```python
from build123d import *

# Parameters (mm, degrees)
F0_R           = 4.7625
F1_DEPTH       = 19.05
F2_R           = 1.8288
F3_DEPTH       = 2.38125
F4_R           = 1.35255
F5_DEPTH       = 2.38125
F8_DEPTH       = 1.190625
F9_R           = 5.55625
F9_R_2         = 4.7625
F11_DEPTH      = 0.79375
F11_DEPTH_BACK = 19.84375
F12_R          = 1.7272
F13_DEPTH      = 10.0554862042
F15_DEPTH      = 19.05
F16_R          = 2.15265
F17_DEPTH      = 2.38125
F18_R          = 1.190625


with BuildPart() as f1:
    # F0 (on Top) → F1 (new body)
    with BuildSketch(Plane.XY):
        Polygon((-12.7, -13.49375), (12.7, -13.49375), (12.7, -21.43125), (15.08125, -21.43125), (15.08125, -11.1125), (7.14375, -11.1125), (7.14375, 7.3428228204), (2.38125, 7.7594875805), (2.38125, 7.14375), (-2.38125, 7.14375), (-2.38125, 7.7594875805), (-7.14375, 7.3428228204), (-7.14375, -11.1125), (-15.08125, -11.1125), (-15.08125, -21.43125), (-12.7, -21.43125), align=None)
        Circle(F0_R, mode=Mode.SUBTRACT)
    extrude(amount=F1_DEPTH)

    # F2 (on face) → F3 (cut, through all)
    with BuildSketch(Plane.YZ.offset(15.08125)):
        with Locations((-18.25625, 15.875)):
            Circle(F2_R)
        with Locations((-18.25625, 3.175)):
            Circle(F2_R)
    extrude(amount=-F3_DEPTH, mode=Mode.SUBTRACT)

    # F4 (on face) → F5 (cut, through all)
    with BuildSketch(Plane(origin=(-15.08125, 0, 0), x_dir=(0, -1, 0), z_dir=(-1, 0, 0))):
        with Locations((18.25625, 3.175)):
            Circle(F4_R)
        with Locations((18.25625, 15.875)):
            Circle(F4_R)
    extrude(amount=-F5_DEPTH, mode=Mode.SUBTRACT)

    # F7 (on offset) → F8 (join, symmetric)
    with BuildSketch(Plane(origin=(0, 0, 9.525), x_dir=(1, 0, 0), z_dir=(0, 0, -1))):
        Polygon((-15.08125, 11.1125), (-7.14375, -7.3428228204), (-7.14375, 11.1125), align=None)
        Polygon((15.08125, 11.1125), (7.14375, 11.1125), (7.14375, -7.3428228204), align=None)
    extrude(amount=F8_DEPTH, both=True)

    # F9 (on face) → F11 (join, two sides)
    with BuildSketch(Plane(origin=(0, 0, 0), x_dir=(1, 0, 0), z_dir=(0, 0, -1))) as f11_sk:
        Circle(F9_R)
        Circle(F9_R_2, mode=Mode.SUBTRACT)
    extrude(amount=F11_DEPTH)
    extrude(f11_sk.sketch, amount=-F11_DEPTH_BACK)

    # F12 (on face) → F13 (cut, up to face)
    with BuildSketch(Plane.XZ.offset(13.49375)):
        with Locations((0, 9.525)):
            Circle(F12_R)
    extrude(amount=-F13_DEPTH, mode=Mode.SUBTRACT)

    # F14 (on face) → F15 (cut, through all)
    with BuildSketch(Plane.XY.offset(19.05)):
        with BuildLine():
            Line((-4.7625, -5.3246368714), (-4.7625, -11.1125))
            Line((-4.7625, -11.1125), (4.7625, -11.1125))
            Line((4.7625, -11.1125), (4.7625, -5.3246368714))
            ThreePointArc((4.7625, -5.3246368714), (0, -7.14375), (-4.7625, -5.3246368714))
        make_face()
    extrude(amount=-F15_DEPTH, mode=Mode.SUBTRACT)

    # F16 (on face) → F17 (cut, through all)
    with BuildSketch(Plane.XZ.offset(13.49375)):
        with Locations((0, 9.525)):
            Circle(F16_R)
    extrude(amount=-F17_DEPTH, mode=Mode.SUBTRACT)

    # F18
    f18_edges = [f1.edges().sort_by_distance(p)[0] for p in [
        (7.14375, -11.1125, 4.167187),
        (7.14375, -11.1125, 14.882812),
        (-7.14375, -11.1125, 4.167187),
        (-7.14375, -11.1125, 14.882812),
        (-4.7625, -11.1125, 9.525),
        (4.7625, -11.1125, 9.525),
        (4.7625, -5.324637, 9.525),
        (-4.7625, -5.324637, 9.525),
    ]]
    fillet(f18_edges, radius=F18_R)


solid = f1.part
```
Check sheet for the modelled part. Datum: model origin and axes. Units: mm. A direction names the side the tool comes from. Round coordinates to 2 decimals unless told otherwise and drop trailing zeros. Loops run counter-clockwise (first coordinate to the right, second up) from the corner with the lowest first, then second, coordinate; pieces in that order, holes last. Notation, with made-up numbers: (-12, 64.25) - (13, 64.25) arc R10 ccw to (13, 83.25) - close; hole circle Ø5 at (89.5, 33.5). An arc over 180 degrees is marked (long way). Write item = value, one per line. Start each with the question number.
Q1. Depth check by flat-ended pin: P1, Ø4, axis at x = -9.5, y = -3, coming from the -Z side; P2, Ø6, axis at y = -6.5, z = 2, coming from the +X side; P3, Ø12, axis at x = 11.5, y = -13.5, coming from the +Z side. Enter the tip coordinate at first touch or a pass-through.
Q2. Section check A-A (x = 0). Record the boundary of the cut face in (y, z).
Q3. Section check C-C (z = 13.5). Record the boundary of the cut face in (x, y) (1 decimal), plus the area to 3 significant figures.
Q4. Section check D-D (x = -4). Record the boundary of the cut face in (y, z), plus the area to 3 significant figures.
Q5. Thickness scan on L1, parallel to X at y = -19.5, z = 13.75; L2, parallel to Y at x = 4, z = 7.25; L3, parallel to X at y = -0.25, z = 17.75. Record the ranges inside material, lowest first.
Q6. Access from +Z, -Z, +X, -X, +Y, -Y to the whole of each face (thin tool, end or side, straight path). Record for faces 5 (the face through (4.194, -6.515, 9.392)), 6 (the face through (-1.273, -5.813, 10.692)), 7 (the face through (-9, -6, 10.716)), 8 (the face through (7.144, -1, 15)), 9 (the face through (7.5, -10.77, 4.23)).
Q7. Section check B-B (y = 1). Record the boundary of the cut face in (x, z).
Q8. Release check for a two-part mould opening along Z. For faces 1 (the face through (5, -2, 19.844)), 2 (the face through (13.907, -20.083, 15.955)), 3 (the face through (4.423, -10.754, 9.392)), 4 (the face through (5, -2, -0.794)) record: pulls with the +Z half, pulls with the -Z half, needs draft (parallel to the pull), parting line crosses it, or undercut.
Derived:
q1.P1 = 8.33
q1.P2 = 7.14
q1.P3 = 19.05
q2.outline = (-13.49, 0) - (-11.11, 0) - (-11.11, 7.37) - (-13.49, 7.37) - close; (-13.49, 11.68) - (-11.11, 11.68) - (-11.11, 19.05) - (-13.49, 19.05) - close; (-7.14, 0) - (-5.56, 0) - (-5.56, -0.79) - (-4.76, -0.79) - (-4.76, 7.8) - (-7.14, 7.8) - close; (-7.14, 11.25) - (-4.76, 11.25) - (-4.76, 19.84) - (-5.56, 19.84) - (-5.56, 19.05) - (-7.14, 19.05) - close; (4.76, -0.79) - (5.56, -0.79) - (5.56, 0) - (7.14, 0) - (7.14, 19.05) - (5.56, 19.05) - (5.56, 19.84) - (4.76, 19.84) - close
q3.outline = (-15.1, -21.4) - (-12.7, -21.4) - (-12.7, -13.5) - (12.7, -13.5) - (12.7, -21.4) - (15.1, -21.4) - (15.1, -11.1) - (8.3, -11.1) arc R1.2 cw to (7.1, -9.9) - (7.1, 7.3) - (2.4, 7.8) - (2.4, 7.1) - (-2.4, 7.1) - (-2.4, 7.8) - (-7.1, 7.3) - (-7.1, -9.9) arc R1.2 cw to (-8.3, -11.1) - (-15.1, -11.1) - close; hole (-4.8, -9.9) arc R1.2 ccw to (-3.6, -11.1) - (3.6, -11.1) arc R1.2 ccw to (4.8, -9.9) - (4.8, -7.5) arc R1.2 ccw to (3.1, -6.5) arc R7.1 cw to (-3.1, -6.5) arc R1.2 ccw to (-4.8, -7.5) - close; hole circle Ø9.5 at (0, 0)
q3.area = 263 mm^2
q4.outline = (-13.49, 0) - (-11.03, 0) - (-11.03, 19.05) - (-13.49, 19.05) - close; (-6.42, 0) - (-3.86, 0) - (-3.86, -0.79) - (-2.58, -0.79) - (-2.58, 19.84) - (-3.86, 19.84) - (-3.86, 19.05) - (-6.42, 19.05) - close; (2.58, -0.79) - (3.86, -0.79) - (3.86, 0) - (7.62, 0) - (7.62, 19.05) - (3.86, 19.05) - (3.86, 19.84) - (2.58, 19.84) - close
q4.area = 220 mm^2
q5.L1 = -15.08 to -12.7, 12.7 to 15.08
q5.L2 = -13.49 to -11.03, -6.42 to -2.58, 2.58 to 7.62
q5.L3 = -7.14 to -4.76, 4.76 to 7.14
q6.face_5 = +Z, -Z
q6.face_6 = -Y
q6.face_7 = +Z, -X, +Y
q6.face_8 = +Z, +X, +Y
q6.face_9 = -Z, +X, +Y
q7.outline = (-9.87, 8.33) - (-7.14, 8.33) - (-7.14, 0) - (-5.47, 0) - (-5.47, -0.79) - (-4.66, -0.79) - (-4.66, 19.84) - (-5.47, 19.84) - (-5.47, 19.05) - (-7.14, 19.05) - (-7.14, 10.72) - (-9.87, 10.72) - close; (4.66, -0.79) - (5.47, -0.79) - (5.47, 0) - (7.14, 0) - (7.14, 8.33) - (9.87, 8.33) - (9.87, 10.72) - (7.14, 10.72) - (7.14, 19.05) - (5.47, 19.05) - (5.47, 19.84) - (4.66, 19.84) - close
q8.face_1 = pulls with the +Z half
q8.face_2 = undercut
q8.face_3 = needs draft
q8.face_4 = pulls with the -Z half
